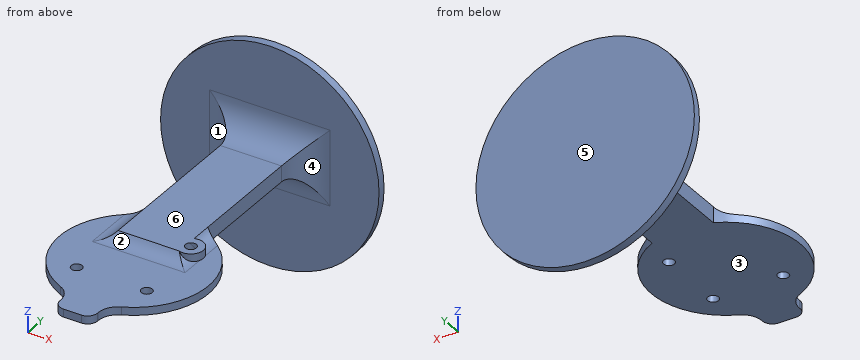
```python
from build123d import *

# Parameters (mm, degrees)
BOSS_EXTRUDE2_DEPTH             = 4
BOSS_EXTRUDE3_DEPTH             = 4
BOSS_EXTRUDE3_DIRECTION_2_REACH = 63.707
FILLET1_R                       = 10
SKETCH4_R                       = 55
BOSS_EXTRUDE4_DEPTH             = 4
FILLET2_R                       = 15
CUT_EXTRUDE1_DEPTH              = 136.949439131
CUT_EXTRUDE1_DEPTH_BACK         = 136.949439131
SKETCH2_4_R                     = 2.75
BOSS_EXTRUDE5_START             = -4
SKETCH5_R                       = 6.283783871
SKETCH5_R_2                     = 2.75
BOSS_EXTRUDE5_DEPTH             = 4


with BuildPart() as part:
    # Sketch2 → Boss-Extrude2 (new body)
    with BuildSketch(Plane.XY):
        with BuildLine():
            Line((-9.448282852, -43.336062282), (-9.448282852, -43.842083491))
            ThreePointArc((-9.448282852, -43.842083491), (-7.983816758, -47.377617397), (-4.448282852, -48.842083491))
            Line((-4.448282852, -48.842083491), (4.448282796, -48.842083491))
            ThreePointArc((4.448282796, -48.842083491), (7.983816702, -47.377617397), (9.448282796, -43.842083491))
            Line((9.448282796, -43.842083491), (9.448282796, -43.336062307))
            ThreePointArc((9.448282796, -43.336062307), (11.053529874, -37.902083712), (15.353907471, -34.212680769))
            ThreePointArc((15.353907471, -34.212680769), (2.4e-08, 37.5), (-15.353907514, -34.212680749))
            ThreePointArc((-15.353907514, -34.212680749), (-11.053529926, -37.902083692), (-9.448282852, -43.336062282))
        make_face()
    extrude(amount=BOSS_EXTRUDE2_DEPTH)

    # Sketch3 → Boss-Extrude3 (add)
    with BuildSketch(Plane.XY.offset(4)):
        with BuildLine():
            Line((-15.37292341, 11.548994525), (15.372923459, 11.548994525))
            Line((15.372923459, 11.548994525), (15.372923459, 34.204140456))
            ThreePointArc((15.372923459, 34.204140456), (2.6e-08, 37.5), (-15.37292341, 34.204140478))
            Line((-15.37292341, 34.204140478), (-15.37292341, 11.548994525))
        make_face()
        with BuildLine():
            ThreePointArc((-15.37292341, 34.204140478), (2.6e-08, 37.5), (15.372923459, 34.204140456))
            Line((15.372923459, 34.204140456), (15.372923459, 107.5))
            Line((15.372923459, 107.5), (-15.37292341, 107.5))
            Line((-15.37292341, 107.5), (-15.37292341, 34.204140478))
        make_face()
    extrude(amount=BOSS_EXTRUDE3_DEPTH)

    # Boss-Extrude3 direction 2: up to this face of the body (flat: up to its plane)
    boss_extrude3_direction_2_end = Plane(part.part.faces().sort_by_distance((-1e-09, -2.077742583, 0))[0])
    # Sketch3 → Boss-Extrude3 direction 2 (add, up to the picked face)
    with BuildSketch(Plane.XY.offset(4), mode=Mode.PRIVATE) as boss_extrude3_direction_2_sk1:
        with BuildLine():
            Line((-15.37292341, 11.548994525), (15.372923459, 11.548994525))
            Line((15.372923459, 11.548994525), (15.372923459, 34.204140456))
            ThreePointArc((15.372923459, 34.204140456), (2.6e-08, 37.5), (-15.37292341, 34.204140478))
            Line((-15.37292341, 34.204140478), (-15.37292341, 11.548994525))
        make_face()
    boss_extrude3_direction_2_tool1 = split(extrude(boss_extrude3_direction_2_sk1.sketch, amount=-BOSS_EXTRUDE3_DIRECTION_2_REACH, mode=Mode.PRIVATE), bisect_by=boss_extrude3_direction_2_end, keep=Keep.BOTH, mode=Mode.PRIVATE)
    # Sketch3 → Boss-Extrude3 direction 2 (add, up to the picked face)
    with BuildSketch(Plane.XY.offset(4), mode=Mode.PRIVATE) as boss_extrude3_direction_2_sk2:
        with BuildLine():
            ThreePointArc((-15.37292341, 34.204140478), (2.6e-08, 37.5), (15.372923459, 34.204140456))
            Line((15.372923459, 34.204140456), (15.372923459, 107.5))
            Line((15.372923459, 107.5), (-15.37292341, 107.5))
            Line((-15.37292341, 107.5), (-15.37292341, 34.204140478))
        make_face()
    boss_extrude3_direction_2_tool2 = split(extrude(boss_extrude3_direction_2_sk2.sketch, amount=-BOSS_EXTRUDE3_DIRECTION_2_REACH, mode=Mode.PRIVATE), bisect_by=boss_extrude3_direction_2_end, keep=Keep.BOTH, mode=Mode.PRIVATE)
    add(boss_extrude3_direction_2_tool1.solids().sort_by(Axis((0, 24.004369, 4), (0, 0, -1)))[0])
    add(boss_extrude3_direction_2_tool2.solids().sort_by(Axis((0, 71.954024, 4), (0, 0, -1)))[0])

    # Fillet1
    # the kernel refuses this fillet: 10 mm, written as the material it adds along each edge
    with BuildSketch(Plane(origin=(-15.37292341, 54.204140478, 4), x_dir=(-1, 0, 0), z_dir=(0, -1, 0))) as fillet1_piece_1_section:
        with BuildLine():
            CenterArc((8, -10), FILLET1_R, 90, 53.130102354)
            Line((0, -4), (-0.16, -3.88))
            ThreePointArc((-0.16, -3.88), (-0.2, -2), (-0.2, 0))
            Line((-0.2, 0), (0, 0.2))
            Line((0, 0.2), (8, 0.2))
            Line((8, 0.2), (8, 0))
        make_face()
    fillet1_piece_1 = extrude(amount=42.655145953, mode=Mode.PRIVATE)
    fillet1_piece_1 = fillet1_piece_1 & Plane(origin=(0, 0, 5.050776903), x_dir=(0.4094375325494367, -0.9123381538332315, 0), z_dir=(0, 0, -1)) * Cylinder(37.5, 118, mode=Mode.PRIVATE)
    add(fillet1_piece_1)
    with BuildSketch(Plane(origin=(-15.37292341, 11.548994525, 4), x_dir=(0, -1, 0), z_dir=(1, 0, 0))) as fillet1_piece_2:
        with BuildLine():
            CenterArc((8, -10), FILLET1_R, 90, 53.130102354)
            Line((0, -4), (-0.16, -3.88))
            ThreePointArc((-0.16, -3.88), (-0.2, -2), (-0.2, 0))
            Line((-0.2, 0), (0, 0.2))
            Line((0, 0.2), (8, 0.2))
            Line((8, 0.2), (8, 0))
        make_face()
    extrude(amount=30.745846869)
    with BuildSketch(Plane(origin=(15.372923459, 54.204140456, 4), x_dir=(1, 0, 0), z_dir=(0, -1, 0))) as fillet1_piece_3_section:
        with BuildLine():
            CenterArc((8, 10), FILLET1_R, 216.869897646, 53.130102354)
            Line((0, 4), (-0.16, 3.88))
            ThreePointArc((-0.16, 3.88), (-0.2, 2), (-0.2, 0))
            Line((-0.2, 0), (0, -0.2))
            Line((0, -0.2), (8, -0.2))
            Line((8, -0.2), (8, 0))
        make_face()
    fillet1_piece_3 = extrude(amount=42.655145931, mode=Mode.PRIVATE)
    fillet1_piece_3 = fillet1_piece_3 & Plane(origin=(0, 0, 5.050777143), x_dir=(0.4094375325494367, -0.9123381538332315, 0), z_dir=(0, 0, -1)) * Cylinder(37.5, 118, mode=Mode.PRIVATE)
    add(fillet1_piece_3)
    with BuildSketch(Plane(origin=(-15.37292341, 54.204140478, 4), x_dir=(-1, 0, 0), z_dir=(0, -1, 0))) as fillet1_piece_4a_section:
        with BuildLine():
            CenterArc((8, -10), FILLET1_R, 90, 53.130102354)
            Line((0, -4), (-0.16, -3.88))
            ThreePointArc((-0.16, -3.88), (-0.2, -2), (-0.2, 0))
            Line((-0.2, 0), (0, 0.2))
            Line((0, 0.2), (8, 0.2))
            Line((8, 0.2), (8, 0))
        make_face()
    fillet1_piece_4a = extrude(amount=62.655145953, mode=Mode.PRIVATE)
    fillet1_piece_4a = split(fillet1_piece_4a, bisect_by=Plane(origin=(-17.431757525, 11.548994525, 5.023885124), z_dir=(0, -1, 0)), keep=Keep.TOP, mode=Mode.PRIVATE)
    with BuildSketch(Plane(origin=(-35.37292341, 11.548994525, 4), x_dir=(0, -1, 0), z_dir=(1, 0, 0))) as fillet1_piece_4b_section:
        with BuildLine():
            CenterArc((8, -10), FILLET1_R, 90, 53.130102354)
            Line((0, -4), (-0.16, -3.88))
            ThreePointArc((-0.16, -3.88), (-0.2, -2), (-0.2, 0))
            Line((-0.2, 0), (0, 0.2))
            Line((0, 0.2), (8, 0.2))
            Line((8, 0.2), (8, 0))
        make_face()
    fillet1_piece_4b = extrude(amount=50.745846869, mode=Mode.PRIVATE)
    fillet1_piece_4b = split(fillet1_piece_4b, bisect_by=Plane(origin=(-15.37292341, 9.490160411, 5.023885124), z_dir=(-1, 0, 0)), keep=Keep.TOP, mode=Mode.PRIVATE)
    fillet1_piece_4 = fillet1_piece_4a & fillet1_piece_4b
    add(fillet1_piece_4)
    with BuildSketch(Plane(origin=(-15.37292341, 11.548994525, 4), x_dir=(0, -1, 0), z_dir=(1, 0, 0))) as fillet1_piece_5a_section:
        with BuildLine():
            CenterArc((8, -10), FILLET1_R, 90, 53.130102354)
            Line((0, -4), (-0.16, -3.88))
            ThreePointArc((-0.16, -3.88), (-0.2, -2), (-0.2, 0))
            Line((-0.2, 0), (0, 0.2))
            Line((0, 0.2), (8, 0.2))
            Line((8, 0.2), (8, 0))
        make_face()
    fillet1_piece_5a = extrude(amount=50.745846869, mode=Mode.PRIVATE)
    fillet1_piece_5a = split(fillet1_piece_5a, bisect_by=Plane(origin=(15.372923459, 9.490160411, 5.023885124), z_dir=(1, 0, 0)), keep=Keep.TOP, mode=Mode.PRIVATE)
    with BuildSketch(Plane(origin=(15.372923459, 54.204140456, 4), x_dir=(1, 0, 0), z_dir=(0, -1, 0))) as fillet1_piece_5b_section:
        with BuildLine():
            CenterArc((8, 10), FILLET1_R, 216.869897646, 53.130102354)
            Line((0, 4), (-0.16, 3.88))
            ThreePointArc((-0.16, 3.88), (-0.2, 2), (-0.2, 0))
            Line((-0.2, 0), (0, -0.2))
            Line((0, -0.2), (8, -0.2))
            Line((8, -0.2), (8, 0))
        make_face()
    fillet1_piece_5b = extrude(amount=62.655145931, mode=Mode.PRIVATE)
    fillet1_piece_5b = split(fillet1_piece_5b, bisect_by=Plane(origin=(17.431757573, 11.548994525, 5.023885124), z_dir=(0, -1, 0)), keep=Keep.TOP, mode=Mode.PRIVATE)
    fillet1_piece_5 = fillet1_piece_5a & fillet1_piece_5b
    add(fillet1_piece_5)

    # Sketch4 → Boss-Extrude4 (add)
    with BuildSketch(Plane(origin=(0, 107.5, 0), x_dir=(1, 0, 0), z_dir=(0, 1, 0))):
        with Locations(Location((0, 0, 0), (0, 0, 270))):
            Circle(SKETCH4_R)
    extrude(amount=BOSS_EXTRUDE4_DEPTH)

    # Fillet2
    fillet2_edges = [part.edges().sort_by_distance(p)[0] for p in [
        (15.372923459, 107.5, 4),
        (-15.37292341, 107.5, 4),
        (2.4e-08, 107.5, 0),
        (2.4e-08, 107.5, 8),
    ]]
    fillet(fillet2_edges, radius=FILLET2_R)

    # Sketch2<4> → Cut-Extrude1 (cut, two sides: drawn at the far end of the back side and taken through both)
    with BuildSketch(Plane.XY.offset(-CUT_EXTRUDE1_DEPTH_BACK)):
        with Locations((17.525184131, 17.452697917)):
            Circle(SKETCH2_4_R)
        with Locations((17.525184131, -17.473883919)):
            Circle(SKETCH2_4_R)
        with Locations((-17.804632122, -17.473883919)):
            Circle(SKETCH2_4_R)
    extrude(amount=CUT_EXTRUDE1_DEPTH + CUT_EXTRUDE1_DEPTH_BACK, mode=Mode.SUBTRACT)

    # Sketch5 → Boss-Extrude5 (add)
    with BuildSketch(Plane.XY.offset(8).offset(BOSS_EXTRUDE5_START)):
        with Locations((17.525184131, 17.452697917)):
            Circle(SKETCH5_R)
        with Locations((17.525184131, 17.452697917)):
            Circle(SKETCH5_R_2, mode=Mode.SUBTRACT)
    extrude(amount=BOSS_EXTRUDE5_DEPTH)


solid = part.part
```
Can you work these out from the model? Positions are in its coordinate system, mm. Face numbers are marked on the shaded views. A direction names the side the tool comes from. Coordinates: 2 decimals unless noted, no trailing zeros. Loops run counter-clockwise (first coordinate to the right, second up) from the corner with the lowest first, then second, coordinate; pieces in that order, holes last. Notation, with made-up numbers: (38.5, -15) -> (62.5, -15) arc R26 ccw to (62.5, 19) -> close; hole circle Ø9 at (-36, -39.5). An arc over 180 degrees is marked (long way). Put each result on its own line as item: value. Start each with the question number.
Q1. I want a section at A-A (x = 34). Write out the boundary of the cut face in (y, z), plus the area to 3 significant figures.
Q2. If I drill on line 1 (Y direction, x = 49, z = 19); line 2 (Z direction, x = -11, y = 32); line 3 (Z direction, x = -2, y = -24.5), over which ranges is the centre line in solid material (lowest first)? Write a range as [from, to].
Q3. I want a section at C-C (y = 76). Write out the boundary of the cut face in (x, z).
Q4. I want a section at B-B (x = 0). Write out the boundary of the cut face in (y, z), plus the area to 3 significant figures.
Q5. Thinking about a two-plate mould opening in Y: for the marked faces 1, 2 and 3, which applies, pulls with the +Y half, pulls with the -Y half, needs draft (parallel to the pull), parting line crosses it, or undercut?
Q6. For the marked faces 4, 5 and 6, which set-ups out of +Z, -Z, +X, -X, +Y, -Y let a thin tool reach every point of the face, with its end or its side?
Q7. I'm going to push flat-ended pins straight in: P1, Ø3.5, axis at x = 17.53, y = 17.45, coming from the -Z side; P2, Ø3, axis at x = 19, y = -21, coming from the +Z side; P3, Ø0.6, axis at y = -43.5, z = 1.5, coming from the -X side; P4, Ø3, axis at x = 40.5, z = 19, coming from the -Y side. Where does each tip first touch, or does it pass through?
Q8. I want a section at D-D (z = 17). Write out the boundary of the cut face in (x, y), plus the area to 3 significant figures.
Taken from the geometry:
1. outline: (-15.82, 0) -> (15.82, 0) -> (15.82, 4) -> (-15.82, 4) -> close; (107.5, -43.23) -> (111.5, -43.23) -> (111.5, 43.23) -> (107.5, 43.23) -> close
1. area: 472 mm2
2. line 1: y = [107.5, 111.5]
2. line 2: z = [0, 8]
2. line 3: z = [0, 4]
3. outline: (-15.37, 0) -> (15.37, 0) -> (15.37, 8) -> (-15.37, 8) -> close
4. outline: (-48.84, 0) -> (92.5, 0) arc R15 cw to (107.5, -15) -> (107.5, -55) -> (111.5, -55) -> (111.5, 55) -> (107.5, 55) -> (107.5, 23) arc R15 cw to (92.5, 8) -> (11.55, 8) arc R10 cw to (3.55, 4) -> (-48.84, 4) -> close
4. area: 1,560 mm2
5. face 1: undercut
5. face 2: pulls with the -Y half
5. face 3: needs draft
6. face 4: +Z, -Z, +X
6. face 5: +Z, -Z, +X, -X, +Y
6. face 6: +Z, +X, -X, -Y
7. P1: passes through
7. P2: stops at z = 4
7. P3: stops at x = -9.45
7. P4: stops at y = 107.5
8. outline: (-52.31, 107.5) -> (-30.37, 107.5) arc R15 cw to (-24.37, 106.25) -> (24.37, 106.25) arc R15 cw to (30.37, 107.5) -> (52.31, 107.5) -> (52.31, 111.5) -> (-52.31, 111.5) -> close
8. area: 484 mm2
